Could you check a few things on this model? Use its own coordinates, in mm. Give positions to 0.01 mm unless a question says otherwise; leave off trailing zeros. Order: outer loops, then holes, each group sorted by start corner. A loop starts at its lowest first (then second) coordinate and runs counter-clockwise, first axis right, second up.
from build123d import *

# Parameters (mm, degrees)
SKETCH1_W           = 80
SKETCH1_H           = 23
SKETCH1_R           = 1.5875
BOSS_EXTRUDE1_DEPTH = 3
SKETCH1_3_W         = 82
SKETCH1_3_H         = 25
SKETCH1_3_W_2       = 80
SKETCH1_3_H_2       = 23
BOSS_EXTRUDE2_DEPTH = 4


with BuildPart() as part:
    # Sketch1 → Boss-Extrude1 (new body)
    with BuildSketch(Plane(origin=(0, 0, 0), x_dir=(1, 0, 0), z_dir=(0, 1, 0))):
        with Locations((40, 11.5)):
            Rectangle(SKETCH1_W, SKETCH1_H)
        with Locations((77.4125, 11.5)):
            Circle(SKETCH1_R, mode=Mode.SUBTRACT)
        with Locations((2.5875, 11.5)):
            Circle(SKETCH1_R, mode=Mode.SUBTRACT)
        with BuildLine():
            ThreePointArc((2, 15.039067674), (6.175, 11.5), (2, 7.960932326))
            Line((2, 7.960932326), (2, 2))
            Line((2, 2), (78, 2))
            Line((78, 2), (78, 7.960932326))
            ThreePointArc((78, 7.960932326), (73.825, 11.5), (78, 15.039067674))
            Line((78, 15.039067674), (78, 21))
            Line((78, 21), (2, 21))
            Line((2, 21), (2, 15.039067674))
        make_face(mode=Mode.SUBTRACT)
    extrude(amount=BOSS_EXTRUDE1_DEPTH)

    # Sketch1_3 → Boss-Extrude2 (add)
    with BuildSketch(Plane(origin=(0, 0, 0), x_dir=(1, 0, 0), z_dir=(0, 1, 0))):
        with Locations((40, 11.5)):
            Rectangle(SKETCH1_3_W, SKETCH1_3_H)
        with Locations((40, 11.5)):
            Rectangle(SKETCH1_3_W_2, SKETCH1_3_H_2, mode=Mode.SUBTRACT)
    extrude(amount=BOSS_EXTRUDE2_DEPTH)


solid = part.part
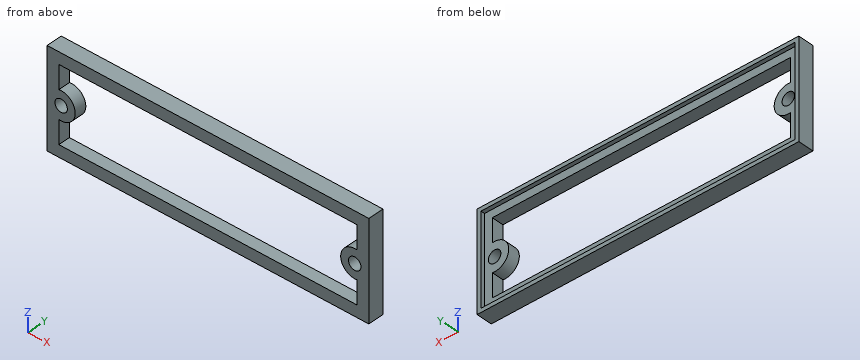
Item 1: Imagine slicing it at B-B on z = -4.25. List the corners of the cut face in (x, y) for me.
Findings:
outline: (-1, 0) - (2, 0) - (2, 3) - (0, 3) - (0, 4) - (-1, 4) - close; (78, 0) - (81, 0) - (81, 4) - (80, 4) - (80, 3) - (78, 3) - close
Item 2: Imagine slicing it at D-D on z = -11.5. List the corners of the cut face in (x, y) for me (3 decimals).
Findings:
outline: (-1, 0) - (1, 0) - (1, 3) - (0, 3) - (0, 4) - (-1, 4) - close; (4.175, 0) - (6.175, 0) - (6.175, 3) - (4.175, 3) - close; (73.825, 0) - (75.825, 0) - (75.825, 3) - (73.825, 3) - close; (79, 0) - (81, 0) - (81, 4) - (80, 4) - (80, 3) - (79, 3) - close
Item 3: Imagine slicing it at C-C on y = 0.95. List the corners of the cut face in (x, z) for me (1 decimal), then the cut area to 3 significant figures.
Findings:
outline: (-1, -24) - (81, -24) - (81, 1) - (-1, 1) - close; hole circle Ø3.2 at (2.6, -11.5); hole (2, -21) - (78, -21) - (78, -15) arc R3.6 cw (long way) to (78, -8) - (78, -2) - (2, -2) - (2, -8) arc R3.6 cw (long way) to (2, -15) - close; hole circle Ø3.2 at (77.4, -11.5)
area: 639 mm2
Item 4: Imagine slicing it at A-A on x = 66. List the corners of the cut face in (y, z) for me, then the cut area to 3 significant figures.
Findings:
outline: (0, -24) - (4, -24) - (4, -23) - (3, -23) - (3, -21) - (0, -21) - close; (0, -2) - (3, -2) - (3, 0) - (4, 0) - (4, 1) - (0, 1) - close
area: 20.0 mm2
Item 5: Please list where these lines run through material, in increasing order: line 1 along X through (y, z) = (0.45, -18.25); line 2 along X through (y, z) = (3.2, -11); line 3 along Z through (x, y) = (39, 3.7).
Findings:
line 1: x = -1 to 2, 78 to 81
line 2: x = -1 to 0, 80 to 81
line 3: z = -24 to -23, 0 to 1
